Autodesk Inventor part; units mm, degrees
ref_plane "YZ Plane" through (0, 0, 0) normal (1, 0, 0) x (0, 1, 0)
ref_plane "XZ Plane" through (0, 0, 0) normal (0, 1, 0) x (-1, 0, 0)
ref_plane "XY Plane" through (0, 0, 0) normal (0, 0, 1) x (1, 0, 0)
sketch "Skizze1" plane through (0, 0, 0) normal (1, 0, 0) x (0, 1, 0)
  line L0 (-21, -18) -> (21, -18)
  line L1 (21, -18) -> (21, 18)
  line L2 (21, 18) -> (-21, 18)
  line L3 (-21, 18) -> (-21, -18)
  line L4 (-21, -18) -> (21, 18) construction
  line L5 (21, -18) -> (-21, 18) construction
  point P0 (0, 0)
  dimension "d0" = 42
  dimension "d1" = 36
extrude "Extrusion1" add sketch "Skizze1" along normal blind 26
fillet "Rundung1" radius 18 2 edges at (13, 21, 18) (13, 21, -18)
sketch "Skizze2" plane through (26, 0, 0) normal (1, 0, 0) x (0, 0, -1)
  arc A0 (18, 3) -> (-18, 3) centre (0, 3) ccw
  circle A1 centre (0, 3) radius 15
  point P0 (0, 0)
  dimension "d5" = 30
hole "Bohrung1" at (26, 3, 0) direction (-1, 0, 0) diameter 30 end through all
ref_plane "Arbeitsebene2" through (0, -18, -18) normal (0, -1, 0) x (1, 0, 0)
ref_plane "Arbeitsebene3" through (0, -14.8, -18) normal (0, -1, 0) x (1, 0, 0)
sketch "Skizze3" plane through (0, -21, -18) normal (0, -1, 0) x (1, 0, 0)
  line L0 (0, 0) -> (26, 0)
  line L1 (3, 0) -> (23, 0)
  line L2 (23, 0) -> (23, 25)
  line L3 (23, 25) -> (3, 25)
  line L4 (3, 25) -> (3, 0)
  point P0 (0, 18)
  point P1 (13, 0)
  dimension "d15" = 20
  dimension "d16" = 25
extrude "Extrusion2" cut sketch "Skizze3" against normal up to surface (3.2 mm away) from surface at -3
fillet "Rundung2" radius 9 2 edges at (23, -16.4, 7) (3, -16.4, 7)
ref_plane "Arbeitsebene7" through (-35.1228, -11.2, 0) normal (0, -1, 0) x (1, 0, 0)
ref_plane "Arbeitsebene6" through (-35.1228, -12, 0) normal (0, -1, 0) x (1, 0, 0)
sketch "Skizze9" plane through (-35.1228, -11.2, 0) normal (0, -1, 0) x (1, 0, 0)
  line L0 (61.1228, 15) -> (61.1228, -15)
  line L1 (61.1228, -18) -> (35.1228, -18)
  point P0 (35.1228, 0)
  point P1 (48.1228, 0)
  dimension "d49" = 13
  dimension "d50" = 18
hole "Bohrung5" at (13, -11.2, 0) direction (0, -1, 0) diameter 4.2 depth 15 countersink diameter 10 countersink angle 90
Build history of the part. All positions in model axes, mm. A direction names the side the tool comes from. Coordinates: 2 decimals unless noted, no trailing zeros. Order: outer loops, then holes, each group sorted by start corner. A loop starts at its lowest first (then second) coordinate and runs counter-clockwise, first axis right, second up. Notation, with made-up numbers: (29.5, 79.5) -> (65.5, 79.5) arc R20 cw to (65.5, 117.5) -> close; hole circle Ø9 at (64.5, -24.75). An arc over 180 degrees is marked (long way). Answer in a Markdown table with one row per item. Add a question column.
Q1. Which spindle directions (+Z, -Z, +X, -X, +Y, -Y) get a long thin tool onto all of the face, cutting with end or side? Do faces 1 (the face through (10.918, -14.455, -0.273)), 2 (the face through (10.976, -13.919, 1.053)), 3 (the face through (23, -16, -10)). Say none if no direction does.
Q2. Band-saw the part on C-C, the plane z = 11. List the corners of the cut face in (x, y), then the cut area to 3 significant figures.
Q3. Drop flat-ended pins along their axis: pin 1 (8 mm diameter, centred on y = 16, z = 6, fed in from +X); pin 2 (1 mm diameter, centred on x = 13.5, y = -16.5, fed in from -Z); pin 3 (4 mm diameter, centred on x = 4, y = 12.5, fed in from +Z); pin 4 (1 mm diameter, centred on x = 11.5, z = -3, fed in from +Y). Give the stop position or say it passes through.
Q4. Wall check: line 1 along Y through (x, z) = (21.25, 0); line 2 along Z through (x, y) = (13, -18.7); line 3 along Y through (x, z) = (5, -3). Give the ranges that are in metal, low to high. Write a range as [from, to].
Q5. Band-saw the part on A-A, the plane z = -12.5. List the corners of the cut face in (x, y), then the cut area to 3 significant figures.
Q6. Mould opens along X. For faces 4 (the face through (13, -9, -18)), 5 (the face through (26, -14, 0)), 6 (the face through (0, -14, 0)), 7 (the face through (13, -18, -5)) say: +X half, -X half, draft (parallel to the pull), parting line (faces both ways), or undercut.
Answers follow:
| question | item | result |
|---|---|---|
| 1 | face 1 | -Y |
| 1 | face 2 | none |
| 1 | face 3 | -Z |
| 2 | outline | (0, -21) -> (26, -21) -> (26, -7.2) -> (0, -7.2) -> close; (0, 13.2) -> (26, 13.2) -> (26, 17.25) -> (0, 17.25) -> close |
| 2 | area | 464 mm^2 |
| 3 | pin 1 | x = 26 |
| 3 | pin 2 | z = 7 |
| 3 | pin 3 | z = 16.36 |
| 3 | pin 4 | y = 20.83 |
| 4 | line 1 | [-21, -18], [-14.8, -12], [18, 21] |
| 4 | line 2 | [-18, -2.1], [2.1, 18] |
| 4 | line 3 | [-21, -18], [-14.8, -11.7], [17.7, 20.75] |
| 5 | outline | (0, -21) -> (26, -21) -> (26, -5.29) -> (0, -5.29) -> close; (0, 11.29) -> (26, 11.29) -> (26, 15.95) -> (0, 15.95) -> close; hole (3, -18) -> (23, -18) -> (23, -14.8) -> (3, -14.8) -> close |
| 5 | area | 466 mm^2 |
| 6 | face 4 | draft |
| 6 | face 5 | +X half |
| 6 | face 6 | -X half |
| 6 | face 7 | undercut |
